Geometry check sheet. Reference: the model listing, model coordinates, mm. A direction names the side the tool comes from. Round coordinates to 2 decimals unless told otherwise and drop trailing zeros. Loops run counter-clockwise (first coordinate to the right, second up) from the corner with the lowest first, then second, coordinate; pieces in that order, holes last.
```python
from build123d import *

# Parameters (mm, degrees)
CUT_EXTRUDE1_DEPTH = 2.5
CHAMFER1_SIZE      = 1


with BuildPart() as part:
    # Sketch1 → Revolve1 (revolve)
    with BuildSketch(Plane(origin=(0, 0, 0), x_dir=(1, 0, 0), z_dir=(0, 1, 0)), mode=Mode.PRIVATE) as revolve1_sk:
        Polygon((-59, 0), (-59, -5), (0, -5), (0, -9), (3, -9), (3, -5), (51, -5), (51, 0), align=None)
    revolve(revolve1_sk.sketch.rotate(Axis((0, 0, 0), (-1, 0, 0)), 180), axis=Axis((0, 0, 0), (-1, 0, 0)))

    # Sketch2 → Cut-Extrude1 (cut)
    with BuildSketch(Plane.XY.offset(5)):
        with BuildLine():
            Line((9, 2), (25, 2))
            ThreePointArc((25, 2), (27, 0), (25, -2))
            Line((25, -2), (9, -2))
            ThreePointArc((9, -2), (7, 0), (9, 2))
        make_face()
    extrude(amount=-CUT_EXTRUDE1_DEPTH, mode=Mode.SUBTRACT)

    # Chamfer1
    chamfer1_edges = [part.edges().sort_by_distance(p)[0] for p in [
        (51, 0, 5),
        (-59, 0, 5),
    ]]
    chamfer(chamfer1_edges, length=CHAMFER1_SIZE)


solid = part.part
```
1) Access from +Z, -Z, +X, -X, +Y, -Y to the whole of each face (thin tool, end or side, straight path). Record for faces 4 (the face through (3, 4, -4)), 5 (the face through (27, 0, 4)), 6 (the face through (51, 0, 0)), 7 (the face through (0, 4, 4)).
Report:
face 4: +X
face 5: +Z
face 6: +Z, -Z, +X, +Y, -Y
face 7: -X
2) Sectioned sample at C-C, the plane x = 40. Record the cut outline in (y, z).
Report:
outline: circle Ø10 at (0, 0)
3) Mould release check, pull along Y, two halves, no side actions. Record for faces 1 (the face through (1.521, -6.083, 6.633)), 2 (the face through (-59, 0, 0)), 3 (the face through (17, 2, 4)): +Y half, -Y half, draft (parallel to the pull), parting line (faces both ways), or undercut.
Report:
face 1: parting line
face 2: draft
face 3: undercut
4) Scan lines: line 1 along X through (y, z) = (3.75, -3.75); line 2 along Y through (x, z) = (-30, 0); line 3 along Y through (x, z) = (15.5, 3). Record each from-to range of solid material in increasing order.
Report:
line 1: x = 0 to 3
line 2: y = -5 to 5
line 3: y = -4 to -2, 2 to 4
5) Gauge pin test, flat ends, axial feed: pin 1 (5 mm diameter, centred on y = 4.5, z = -5, fed in from +X); pin 2 (2 mm diameter, centred on x = -8.5, z = 2.5, fed in from -Y); pin 3 (4 mm diameter, centred on y = 2.5, z = -4, fed in from -X); pin 4 (1 mm diameter, centred on x = 20.5, z = 4, fed in from -Y). Record the tip position at first contact, or that the pin passes through.
Report:
pin 1: stops at x = 50.77
pin 2: stops at y = -4.77
pin 3: stops at x = -59
pin 4: stops at y = -3.57
6) Sectioned sample at B-B, the plane y = 6.5. Record the cut outline in (x, z).
Report:
outline: (0, -6.22) - (3, -6.22) - (3, 6.22) - (0, 6.22) - close
7) Sectioned sample at A-A, the plane x = 23. Record the cut outline in (y, z), then the cut area to 3 significant figures.
Report:
outline: (-2, 2.5) - (-2, 4.58) arc R5 ccw (long way) to (2, 4.58) - (2, 2.5) - close
area: 69.1 mm2
